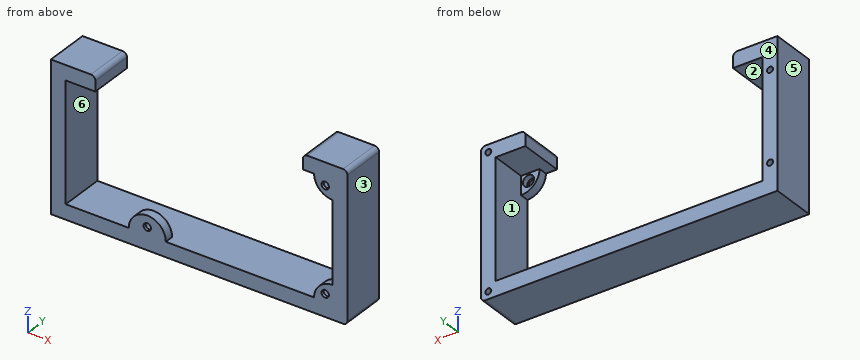
```python
from build123d import *

# Parameters (mm, degrees)
SKETCH1_W           = 200
SKETCH1_H           = 100
SKETCH1_W_2         = 180
SKETCH1_H_2         = 80
BOSS_EXTRUDE1_DEPTH = 30
SKETCH2_R           = 2.5
BOSS_EXTRUDE2_DEPTH = 6
SKETCH3_R           = 3.75
CUT_EXTRUDE1_DEPTH  = 4
SKETCH4_R           = 2
CUT_EXTRUDE2_DEPTH  = 15
SKETCH5_W           = 140
SKETCH5_H           = 10
CUT_EXTRUDE3_DEPTH  = 116.758369028
FILLET1_R           = 3


with BuildPart() as part:
    # Sketch1 → Boss-Extrude1 (new body)
    with BuildSketch(Plane(origin=(0, 0, 0), x_dir=(1, 0, 0), z_dir=(0, 1, 0))):
        Rectangle(SKETCH1_W, SKETCH1_H)
        Rectangle(SKETCH1_W_2, SKETCH1_H_2, mode=Mode.SUBTRACT)
    extrude(amount=BOSS_EXTRUDE1_DEPTH)

    # Sketch2 → Boss-Extrude2 (add)
    # profile 1 of 3: a face of its own
    with BuildSketch(Plane(origin=(0, 0, 0), x_dir=(1, 0, 0), z_dir=(0, 1, 0))):
        with BuildLine():
            Line((77.5, 40), (90, 40))
            Line((90, 40), (90, 27.5))
            ThreePointArc((90, 27.5), (81.161165235, 31.161165235), (77.5, 40))
        make_face()
        with Locations(Location((85, 35, 0), (0, 0, 270))):
            Circle(SKETCH2_R, mode=Mode.SUBTRACT)
    # profile 2 of 3: a face of its own
    with BuildSketch(Plane(origin=(0, 0, 0), x_dir=(1, 0, 0), z_dir=(0, 1, 0))):
        with BuildLine():
            Line((90, -40), (90, -27.5))
            ThreePointArc((90, -27.5), (81.161165235, -31.161165235), (77.5, -40))
            Line((77.5, -40), (90, -40))
        make_face()
        with Locations(Location((85, -35, 0), (0, 0, 90))):
            Circle(SKETCH2_R, mode=Mode.SUBTRACT)
    # profile 3 of 3: a face of its own
    with BuildSketch(Plane(origin=(0, 0, 0), x_dir=(1, 0, 0), z_dir=(0, 1, 0))):
        with BuildLine():
            Line((-47.5, 40), (-22.5, 40))
            ThreePointArc((-22.5, 40), (-35, 27.5), (-47.5, 40))
        make_face()
        with Locations(Location((-35, 35, 0), (0, 0, 270))):
            Circle(SKETCH2_R, mode=Mode.SUBTRACT)
    extrude(amount=BOSS_EXTRUDE2_DEPTH)

    # Sketch3 → Cut-Extrude1 (cut)
    with BuildSketch(Plane(origin=(0, 6, 0), x_dir=(1, 0, 0), z_dir=(0, 1, 0))):
        with Locations(Location((-35, 35, 0), (0, 0, 270))):
            Circle(SKETCH3_R)
        with Locations(Location((85, 35, 0), (0, 0, 270))):
            Circle(SKETCH3_R)
        with Locations(Location((85, -35, 0), (0, 0, 90))):
            Circle(SKETCH3_R)
    extrude(amount=-CUT_EXTRUDE1_DEPTH, mode=Mode.SUBTRACT)

    # Sketch4 → Cut-Extrude2 (cut)
    with BuildSketch(Plane(origin=(0, 30, 0), x_dir=(1, 0, 0), z_dir=(0, 1, 0))):
        with Locations(Location((95, 45, 0), (0, 0, 270))):
            Circle(SKETCH4_R)
        with Locations(Location((95, -45, 0), (0, 0, 90))):
            Circle(SKETCH4_R)
        with Locations(Location((-95, 30, 0), (0, 0, 270))):
            Circle(SKETCH4_R)
        with Locations(Location((-95, -30, 0), (0, 0, 90))):
            Circle(SKETCH4_R)
    extrude(amount=-CUT_EXTRUDE2_DEPTH, mode=Mode.SUBTRACT)

    # Sketch5 → Cut-Extrude3 (cut, through all)
    with BuildSketch(Plane(origin=(0, 30, 0), x_dir=(1, 0, 0), z_dir=(0, 1, 0))):
        with Locations((0, -45)):
            Rectangle(SKETCH5_W, SKETCH5_H)
    extrude(amount=-CUT_EXTRUDE3_DEPTH, mode=Mode.SUBTRACT)

    # Fillet1
    fillet1_edges = [part.edges().sort_by_distance(p)[0] for p in [
        (70, 15, 50),
        (-70, 15, 50),
        (100, 15, 50),
        (100, 15, -50),
    ]]
    fillet(fillet1_edges, radius=FILLET1_R)


solid = part.part
```
Read the model definition and answer for the solid it produces. Units are mm, in the model's axes. Face numbers are marked on the shaded views. A direction names the side the tool comes from. Coordinates: 2 decimals unless noted, no trailing zeros. Loops run counter-clockwise (first coordinate to the right, second up) from the corner with the lowest first, then second, coordinate; pieces in that order, holes last. Notation, with made-up numbers: (42, 32) -> (60, 32) arc R9 cw to (60, 46) -> close; hole circle Ø2 at (-13.5, 23.25). An arc over 180 degrees is marked (long way). Return JSON: item names as keys, results as strings.
Item 1: Find section B-B (x = -35). Determine the outline of the cut face in (y, z).
Answers:
{"outline": "(0, -50) -> (30, -50) -> (30, -40) -> (6, -40) -> (6, -38.75) -> (2, -38.75) -> (2, -37.5) -> (0, -37.5) -> close; (0, -32.5) -> (2, -32.5) -> (2, -31.25) -> (6, -31.25) -> (6, -27.5) -> (0, -27.5) -> close"}
Item 2: Find section C-C (z = -20.5). Determine the outline of the cut face in (x, y).
Answers:
{"outline": "(-100, 0) -> (-90, 0) -> (-90, 30) -> (-100, 30) -> close; (90, 0) -> (100, 0) -> (100, 30) -> (90, 30) -> close"}
Item 3: Find section D-D (x = -95). Determine the outline of the cut face in (y, z).
Answers:
{"outline": "(0, -50) -> (30, -50) -> (30, -32) -> (15, -32) -> (15, -28) -> (30, -28) -> (30, 28) -> (15, 28) -> (15, 32) -> (30, 32) -> (30, 50) -> (0, 50) -> close"}
Item 4: For the marked faces 1, 2 and 3, determine the directions among +Z, -Z, +X, -X, +Y, -Y from which every point of the face is accessible in a straight line to the end or side of a thin tool.
Answers:
{"face 1": "+Y", "face 2": "+Y, -Y", "face 3": "+Z, -Z, +X, +Y, -Y"}
Item 5: For a pull along X with two mould halves and no side action, classify the marked faces 4, 5 and 6 as +X half, -X half, draft (parallel to the pull), parting line (faces both ways), or undercut.
Answers:
{"face 4": "draft", "face 5": "-X half", "face 6": "undercut"}
Item 6: Find section A-A (y = 21.5). Determine the outline of the cut face in (x, z).
Answers:
{"outline": "(-100, -50) -> (97, -50) arc R3 ccw to (100, -47) -> (100, 47) arc R3 ccw to (97, 50) -> (73, 50) arc R3 ccw to (70, 47) -> (70, 40) -> (90, 40) -> (90, -40) -> (-90, -40) -> (-90, 40) -> (-70, 40) -> (-70, 47) arc R3 ccw to (-73, 50) -> (-100, 50) -> close; hole circle Ø4 at (-95, -30); hole circle Ø4 at (-95, 30); hole circle Ø4 at (95, -45); hole circle Ø4 at (95, 45)"}
Item 7: Flat-ended cylindrical pins translate along their axes: P1, Ø2.5, axis at x = -95, z = -30, coming from the +Y side; P2, Ø6, axis at x = 86, z = -36, coming from the +Y side; P3, Ø15, axis at x = -20.5, y = 11.5, coming from the +Z side. Find the tip coordinate at first contact, or state that the pin passes through.
Answers:
{"P1": "stops at y = 15", "P2": "stops at y = 6", "P3": "stops at z = -31.76"}
Item 8: Find the intervals of material crossed by probe 1 along X at (y, z) = (25.5, -30); probe 2 along X at (y, z) = (3, 1); probe 3 along Z at (x, y) = (-35, 0.75), in increasing order.
Answers:
{"probe 1": "x = -100 to -97, -93 to -90, 90 to 100", "probe 2": "x = -100 to -90, 90 to 100", "probe 3": "z = -50 to -37.5, -32.5 to -27.5"}
